Input: dimensioned drawing with shaded views. Units: mm. Origin: part minimum x, y, z. Round coordinates to 2 decimals unless told otherwise and drop trailing zeros. Order: outer loops, then holes, each group sorted by start corner. A loop starts at its lowest first (then second) coordinate and runs counter-clockwise, first axis right, second up. Notation, with made-up numbers: (65, 68.25) - (86, 68.25) arc R21 cw to (86, 73.25) - close; hole circle Ø2 at (-18.5, 35). An arc over 180 degrees is marked (long way). Put each result on its own line as item: value. Start each with the question number.
(1) Section A-A (z = 72.5). Output: boundary loops of the cut face in (x, y) (3 decimals).
(2) Section B-B (y = 85). Output: boundary loops of the cut face in (x, z) (3 decimals), and give its area (3 significant figures).
(3) Material intervals for L1, parallel to Z at x = 23.5, y = 85 (3 decimals); L2, parallel to Y at x = 3.25, z = 76; L3, parallel to Y at x = 23.25, z = 74, sorted ascending. Write a range as [from, to].
(4) Pin query (flat end, axial travel): P1, Ø7.5, axis at y = 15, z = 72.5, coming from the -X side; P2, Ø5, axis at x = 17, y = 32, coming from the -Z side. Return the tip coordinate at first contact, or that it passes through.
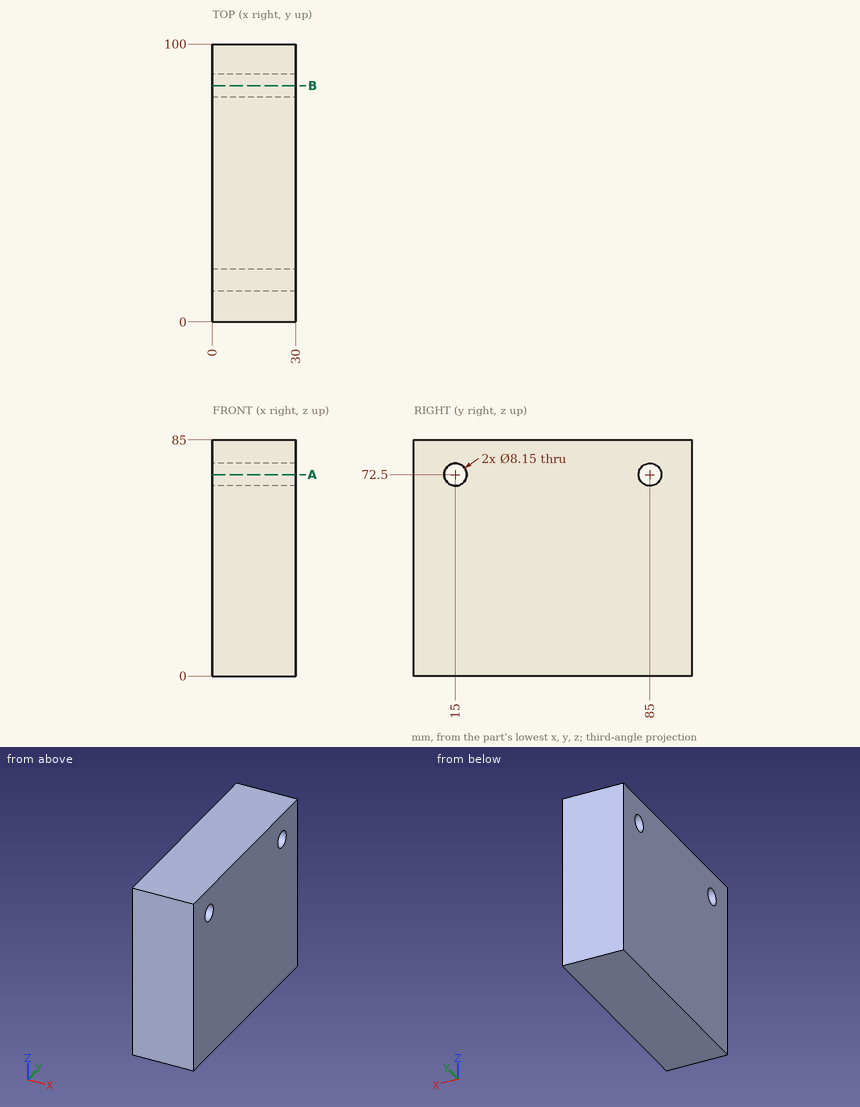
Checks:
1. outline: (0, 0) - (30, 0) - (30, 10.925) - (0, 10.925) - close; (0, 19.075) - (30, 19.075) - (30, 80.925) - (0, 80.925) - close; (0, 89.075) - (30, 89.075) - (30, 100) - (0, 100) - close
2. outline: (0, 0) - (30, 0) - (30, 68.425) - (0, 68.425) - close; (0, 76.575) - (30, 76.575) - (30, 85) - (0, 85) - close
2. area: 2,310 mm²
3. L1: z = [0, 68.425], [76.575, 85]
3. L2: y = [0, 12.91], [17.09, 82.91], [87.09, 100]
3. L3: y = [0, 11.21], [18.79, 81.21], [88.79, 100]
4. P1: passes through
4. P2: stops at z = 0
